from build123d import *

# Parameters (mm, degrees)
BOSS_EXTRUDE1_DEPTH    = 80
SKETCH2_R              = 25
BOSS_EXTRUDE2_DEPTH    = 40
CUT_EXTRUDE2_DEPTH     = 40
M20_TAPPED_HOLE2_D     = 17.5
M20_TAPPED_HOLE2_DEPTH = 30
M20_TAPPED_HOLE2_TIP   = 5.257530416
SKETCH9_W              = 140
SKETCH9_H              = 40
CUT_EXTRUDE3_DEPTH     = 110
M20_TAPPED_HOLE3_D     = 17.5
M20_TAPPED_HOLE3_DEPTH = 37.5
M20_TAPPED_HOLE3_TIP   = 5.257530416
SKETCH14_R             = 25
SKETCH14_R_2           = 15
BOSS_EXTRUDE3_DEPTH    = 30
SKETCH15_R             = 15
BOSS_EXTRUDE4_DEPTH    = 30
SKETCH16_R             = 15
CUT_EXTRUDE4_DEPTH     = 15
M20_TAPPED_HOLE4_D     = 17.5
M20_TAPPED_HOLE4_DEPTH = 60
M20_TAPPED_HOLE4_TIP   = 5.257530416


with BuildPart() as part:
    # Sketch1 → Boss-Extrude1 (new body)
    with BuildSketch(Plane.XY):
        with BuildLine():
            Line((54.268808187, 99.430121053), (4.268808187, 58.948665044))
            ThreePointArc((4.268808187, 58.948665044), (1.121855986, 54.957351344), (0, 50))
            Line((0, 50), (0, 0))
            Line((0, 0), (140, 0))
            Line((140, 0), (140, 50))
            ThreePointArc((140, 50), (138.878144014, 54.957351344), (135.731191813, 58.948665044))
            Line((135.731191813, 58.948665044), (85.731191813, 99.430121053))
            ThreePointArc((85.731191813, 99.430121053), (92.56412856, 90.763833069), (95, 80))
            ThreePointArc((95, 80), (59.236166931, 57.43587144), (54.268808187, 99.430121053))
        make_face()
    extrude(amount=BOSS_EXTRUDE1_DEPTH)

    # Sketch2 → Boss-Extrude2 (add)
    with BuildSketch(Plane(origin=(0, 0, 0), x_dir=(-1, 0, 0), z_dir=(0, 0, -1))):
        with Locations((-70, 80)):
            Circle(SKETCH2_R)
    extrude(amount=-BOSS_EXTRUDE2_DEPTH)

    # Sketch3 → Cut-Extrude2 (cut)
    with BuildSketch(Plane.XY.offset(80)):
        with BuildLine():
            ThreePointArc((54.268808187, 99.430121053), (47.43587144, 90.763833069), (45, 80))
            Line((45, 80), (95, 80))
            ThreePointArc((95, 80), (92.56412856, 90.763833069), (85.731191813, 99.430121053))
            Line((85.731191813, 99.430121053), (95, 91.925824036))
            Line((95, 91.925824036), (95, 118.127818218))
            Line((95, 118.127818218), (45, 118.127818218))
            Line((45, 118.127818218), (45, 91.925824036))
            Line((45, 91.925824036), (54.268808187, 99.430121053))
        make_face()
        with BuildLine():
            Line((45, 91.925824036), (45, 80))
            ThreePointArc((45, 80), (47.43587144, 90.763833069), (54.268808187, 99.430121053))
            Line((54.268808187, 99.430121053), (45, 91.925824036))
        make_face()
        with BuildLine():
            ThreePointArc((85.731191813, 99.430121053), (92.56412856, 90.763833069), (95, 80))
            Line((95, 80), (95, 91.925824036))
            Line((95, 91.925824036), (85.731191813, 99.430121053))
        make_face()
    extrude(amount=-CUT_EXTRUDE2_DEPTH, mode=Mode.SUBTRACT)

    # M20 Tapped Hole2
    with Locations(Plane(origin=(20, 0, 20), x_dir=(0, 0, -1), z_dir=(0, -1, 0))):
        with Locations((0, 0), (0, 100)):
            Hole(M20_TAPPED_HOLE2_D / 2, depth=M20_TAPPED_HOLE2_DEPTH)
            with Locations((0, 0, -(M20_TAPPED_HOLE2_DEPTH + M20_TAPPED_HOLE2_TIP / 2))):  # 118° drill point
                Cone(0, M20_TAPPED_HOLE2_D / 2, M20_TAPPED_HOLE2_TIP, mode=Mode.SUBTRACT)

    # Sketch9 → Cut-Extrude3 (cut)
    with BuildSketch(Plane(origin=(0, 20, 0), x_dir=(1, 0, 0), z_dir=(0, 1, 0))):
        with Locations((70, -60)):
            Rectangle(SKETCH9_W, SKETCH9_H)
    extrude(amount=CUT_EXTRUDE3_DEPTH, mode=Mode.SUBTRACT)

    # M20 Tapped Hole3
    with Locations(Plane(origin=(20, 20, 60), x_dir=(0, 0, 1), z_dir=(0, 1, 0))):
        with Locations((0, 0), (0, 100)):
            Hole(M20_TAPPED_HOLE3_D / 2, depth=M20_TAPPED_HOLE3_DEPTH)
            with Locations((0, 0, -(M20_TAPPED_HOLE3_DEPTH + M20_TAPPED_HOLE3_TIP / 2))):  # 118° drill point
                Cone(0, M20_TAPPED_HOLE3_D / 2, M20_TAPPED_HOLE3_TIP, mode=Mode.SUBTRACT)

    # Sketch14 → Boss-Extrude3 (add)
    with BuildSketch(Plane.XY.offset(40)):
        with Locations(Location((70, 80, 0), (0, 0, 128.994638965))):
            Circle(SKETCH14_R)
        with Locations((70, 80)):
            Circle(SKETCH14_R_2, mode=Mode.SUBTRACT)
    extrude(amount=BOSS_EXTRUDE3_DEPTH)

    # Sketch15 → Boss-Extrude4 (add)
    with BuildSketch(Plane.XY.offset(40)):
        with Locations((70, 80)):
            Circle(SKETCH15_R)
    extrude(amount=BOSS_EXTRUDE4_DEPTH)

    # Sketch16 → Cut-Extrude4 (cut)
    with BuildSketch(Plane.XY.offset(70)):
        with Locations((70, 80)):
            Circle(SKETCH16_R)
    extrude(amount=-CUT_EXTRUDE4_DEPTH, mode=Mode.SUBTRACT)

    # M20 Tapped Hole4
    with Locations(Plane(origin=(70, 80, 55), x_dir=(1, 0, 0), z_dir=(0, 0, 1))):
        with Locations((0, 0)):
            Hole(M20_TAPPED_HOLE4_D / 2, depth=M20_TAPPED_HOLE4_DEPTH)
            with Locations((0, 0, -(M20_TAPPED_HOLE4_DEPTH + M20_TAPPED_HOLE4_TIP / 2))):  # 118° drill point
                Cone(0, M20_TAPPED_HOLE4_D / 2, M20_TAPPED_HOLE4_TIP, mode=Mode.SUBTRACT)


solid = part.part
For this review, take the finished solid that the model builds, in its own axes (mm). A direction names the side the tool comes from. Coordinates: 2 decimals unless noted, no trailing zeros. Write each loop counter-clockwise with the first axis right and the second up, starting at its lowest first coordinate (ties: lowest second). Pieces come first, ordered by that corner, then holes. Notation, with made-up numbers: (14.25, -21.5) -> (73.25, -21.5) arc R27 ccw to (73.25, -3.5) -> close; hole circle Ø4 at (2, 55.25). An arc over 180 degrees is marked (long way). Write each question's results on one line, items separated by ' | '. Start each with the question number.
1) Wall thickness on L1, parallel to Y at x = 70, z = 59.25; L2, parallel to X at y = 8, z = 60; L3, parallel to X at y = 23, z = 24: over which ranges is each line inside the solid? List them lowest first. Write a range as [from, to].
2) Consider section B-B (x = 70). Write out the cut boundary in (y, z), plus the area to 3 significant figures.
3) Consider section A-A (z = 60). Write out the cut boundary in (x, y).
4) Consider section D-D (z = 35). Write out the cut boundary in (x, y).
5) Consider section C-C (y = 82). Write out the cut boundary in (x, z).
6) The part is to be moulded in two halves that separate along X. For faces 4 (the face through (138.91, 54.89, 19.72)), 5 (the face through (71, 42, 0)), 6 (the face through (76.5, 73.5, 55)), say which applies: +X half, -X half, draft (parallel to the pull), parting line (faces both ways), or undercut.
7) Insertion check: pin 1 (4 mm diameter, centred on x = 123.5, z = 64, fed in from +Y); pin 2 (12 mm diameter, centred on x = 44.5, y = 55, fed in from +Z); pin 3 (23 mm diameter, centred on x = 70, y = 80, fed in from +Z); pin 4 (24 mm diameter, centred on x = 63, y = 80, fed in from +Z). Each pin has a flat end and moves straight along its axis. Give the tip position at first contact, or say it passes through.
8) For faces 1 (the face through (27.38, 15.21, 24.7)), 2 (the face through (66.748, 65.357, 62.605)), 3 (the face through (69, 20, 60)), list the 3-axis set-ups (+Z, -Z, +X, -X, +Y, -Y) from which the entire face can be reached by the end or side of a thin tool; tool diameter is ignored.
Geometry says:
1) L1: [0, 20], [55, 65], [95, 105] | L2: [0, 11.25], [28.75, 111.25], [128.75, 140] | L3: [0, 12.22], [27.78, 112.22], [127.78, 140]
2) outline: (0, 0) -> (71.25, 0) -> (71.25, 55) -> (65, 55) -> (65, 70) -> (55, 70) -> (55, 40) -> (20, 40) -> (20, 80) -> (0, 80) -> close; (88.75, 0) -> (105, 0) -> (105, 70) -> (95, 70) -> (95, 55) -> (88.75, 55) -> close | area: 5,090 mm^2
3) outline: (0, 0) -> (11.25, 0) -> (11.25, 20) -> (0, 20) -> close; (28.75, 0) -> (111.25, 0) -> (111.25, 20) -> (28.75, 20) -> close; circle Ø50 at (70, 80); (128.75, 0) -> (140, 0) -> (140, 20) -> (128.75, 20) -> close; hole circle Ø30 at (70, 80)
4) outline: (0, 0) -> (140, 0) -> (140, 50) arc R11.51 ccw to (135.73, 58.95) -> (85.73, 99.43) arc R25 ccw to (54.27, 99.43) -> (4.27, 58.95) arc R11.51 ccw to (0, 50) -> close; hole circle Ø17.5 at (70, 80)
5) outline: (32.74, 0) -> (61.48, 0) -> (61.48, 55) -> (55.13, 55) -> (55.13, 70) -> (45.08, 70) -> (45.08, 40) -> (32.74, 40) -> close; (78.52, 0) -> (107.26, 0) -> (107.26, 40) -> (94.92, 40) -> (94.92, 70) -> (84.87, 70) -> (84.87, 55) -> (78.52, 55) -> close
6) face 4: +X half | face 5: draft | face 6: undercut
7) pin 1: through | pin 2: z = 40 | pin 3: z = 55 | pin 4: z = 70
8) face 1: -Y | face 2: +Z | face 3: +Z, +X, -X
